Geometry check sheet. Reference: the model listing, model coordinates, mm. A direction names the side the tool comes from. Round coordinates to 2 decimals unless told otherwise and drop trailing zeros. Loops run counter-clockwise (first coordinate to the right, second up) from the corner with the lowest first, then second, coordinate; pieces in that order, holes last. Notation, with made-up numbers: M 58.5,7.25 L 83.5,7.25 A23 cw 83.5,20.25 Z; hole C 58,-38.5 d6. An arc over 180 degrees is marked long. Answer in a Markdown table with one row per item. Add a question column.
```python
from build123d import *

# Parameters (mm, degrees)
BOSS_EXTRUDE1_DEPTH = 35


with BuildPart() as part:
    # Sketch1 → Boss-Extrude1 (new body)
    with BuildSketch(Plane(origin=(0, 0, 0), x_dir=(1, 0, 0), z_dir=(0, 1, 0))):
        Polygon((-5.5, -26.5), (5.5, -26.5), (5.5, -2.886751346), (0.5, 0), (-0.5, 0), (-5.5, -2.886751346), align=None)
    extrude(amount=BOSS_EXTRUDE1_DEPTH)

    # Sketch2 → Cut-Revolve1 (revolve, cut)
    with BuildSketch(Plane(origin=(0, 0, 0), x_dir=(0, 0, -1), z_dir=(1, 0, 0))):
        Polygon((-14.5, 35), (-11.55, 35), (-11.55, 6), (-12.9, 6), (-12.9, 1.3), (-12, 1.3), (-12, 0), (-14.5, 0), align=None)
    revolve(axis=Axis((0, 0, 14.5), (0, 1, 0)), mode=Mode.SUBTRACT)

    # Sketch3 → Cut-Revolve2 (revolve, cut)
    with BuildSketch(Plane(origin=(0, 0, 0), x_dir=(0, 0, -1), z_dir=(1, 0, 0))):
        Polygon((-22.5, 35), (-19.55, 35), (-19.55, 6), (-20.9, 6), (-20.9, 1.3), (-20, 1.3), (-20, 0), (-22.5, 0), align=None)
    revolve(axis=Axis((0, 0, 22.5), (0, 1, 0)), mode=Mode.SUBTRACT)


solid = part.part
```
1) Cross-section at A-A, the plane x = 0. Record the boundary of the cut face in (y, z).
2) Go/stop test with flat-tipped pins: pin 1 (1.5 mm diameter, centred on x = 0, z = 22.5, fed in from -Y); pin 2 (3 mm diameter, centred on x = -1.5, y = 31.5, fed in from -Z); pin 3 (4 mm diameter, centred on x = 0, z = 22.5, fed in from +Y); pin 4 (6 mm diameter, centred on x = -4.5, y = 12.5, fed in from -Z). Record where each tip stops, or that it passes through.
3) Draft check along X on faces 4 (the flat face through (1, 6, 21)), 5 (the flat face through (0, 17, 0)), 6 (the flat face through (2, 1.3, 14)), 7 (the flat face through (5.5, 17, 15)). Enter one of: +X half, -X half, draft (parallel to the pull), parting line (faces both ways), or undercut.
4) Cross-section at C-C, the plane z = 14.5. Record the boundary of the cut face in (x, y), plus the area to 3 significant figures.
5) Set-up check for faces 1 (the flat face through (-3, 0, 13)), 2 (the flat face through (2, 1.3, 22)), 3 (the cylindrical face through (-0.886, 20.297, 19.686)): record each of +Z, -Z, +X, -X, +Y, -Y from which the full face is reachable in a straight line by a thin tool's end or side.
6) Cross-section at B-B, the plane y = 24. Record the boundary of the cut face in (x, z).
7) Thickness scan on L1, parallel to Z at x = 0, y = 2.35; L2, parallel to Z at x = 0, y = 33.5; L3, parallel to X at y = 4.45, z = 14.5. Record the ranges inside material, lowest first. Write a range as [from, to].
8) Cross-section at D-D, the plane y = 3.5. Record the boundary of the cut face in (x, z).
Worked answers:
| question | item | result |
|---|---|---|
| 1 | outline | M 0,0 L 35,0 L 35,11.55 L 6,11.55 L 6,12.9 L 1.3,12.9 L 1.3,12 L 0,12 Z; M 0,17 L 1.3,17 L 1.3,16.1 L 6,16.1 L 6,17.45 L 35,17.45 L 35,19.55 L 6,19.55 L 6,20.9 L 1.3,20.9 L 1.3,20 L 0,20 Z; M 0,25 L 1.3,25 L 1.3,24.1 L 6,24.1 L 6,25.45 L 35,25.45 L 35,26.5 L 0,26.5 Z |
| 2 | pin 1 | passes through |
| 2 | pin 2 | stops at z = 0 |
| 2 | pin 3 | stops at y = 6 |
| 2 | pin 4 | stops at z = 0.58 |
| 3 | face 4 | undercut |
| 3 | face 5 | draft |
| 3 | face 6 | undercut |
| 3 | face 7 | +X half |
| 4 | outline | M -5.5,0 L -2.5,0 L -2.5,1.3 L -1.6,1.3 L -1.6,6 L -2.95,6 L -2.95,35 L -5.5,35 Z; M 1.6,1.3 L 2.5,1.3 L 2.5,0 L 5.5,0 L 5.5,35 L 2.95,35 L 2.95,6 L 1.6,6 Z |
| 4 | area | 192 mm2 |
| 5 | face 1 | +Z, -Z, +X, -X, -Y |
| 5 | face 2 | -Y |
| 5 | face 3 | +Y |
| 6 | outline | M -5.5,2.89 L -0.5,0 L 0.5,0 L 5.5,2.89 L 5.5,26.5 L -5.5,26.5 Z; hole C 0,14.5 d5.9; hole C 0,22.5 d5.9 |
| 7 | L1 | z = [0, 12.9], [16.1, 20.9], [24.1, 26.5] |
| 7 | L2 | z = [0, 11.55], [17.45, 19.55], [25.45, 26.5] |
| 7 | L3 | x = [-5.5, -1.6], [1.6, 5.5] |
| 8 | outline | M -5.5,2.89 L -0.5,0 L 0.5,0 L 5.5,2.89 L 5.5,26.5 L -5.5,26.5 Z; hole C 0,14.5 d3.2; hole C 0,22.5 d3.2 |
